The model under review builds one solid part; all positions refer to its coordinate system, in mm. A direction names the side the tool comes from. Coordinates: 2 decimals unless noted, no trailing zeros. Order: outer loops, then holes, each group sorted by start corner. A loop starts at its lowest first (then second) coordinate and runs counter-clockwise, first axis right, second up. Notation, with made-up numbers: M 23,-35.5 L 46,-35.5 A9 ccw 46,-27.5 Z; hole C 48.25,-28 d10. An arc over 180 degrees is marked long. Write each question's results on one line, items separated by ' | '.
from build123d import *

# Parameters (mm, degrees)
SKETCH1_R                 = 2.5
BOSS_EXTRUDE1_DEPTH       = 150
SKETCH3_R                 = 3
BOSS_EXTRUDE2_DEPTH       = 15
SKETCH4_R                 = 2
BOSS_EXTRUDE3_DEPTH       = 8
BOSS_EXTRUDE4_DEPTH       = 4
BOSS_EXTRUDE4_DEPTH_BACK  = 4
SKETCH5_R                 = 2.5
BOSS_EXTRUDE5_START       = 65
BOSS_EXTRUDE5_OUTLINE_R   = 4
BOSS_EXTRUDE5_OUTLINE_R_2 = 2.5
BOSS_EXTRUDE5_DEPTH       = 60


# Read off the part's stored shape, not the designer's step: Boss-Extrude5
with BuildPart() as part:
    # Sketch1 → Boss-Extrude1 (new body)
    with BuildSketch(Plane(origin=(0, 0, 0), x_dir=(0, 0, -1), z_dir=(1, 0, 0))):
        Circle(SKETCH1_R)
    extrude(amount=BOSS_EXTRUDE1_DEPTH)

    # Sketch3 → Boss-Extrude2 (add)
    with BuildSketch(Plane.ZY):
        Circle(SKETCH3_R)
    extrude(amount=BOSS_EXTRUDE2_DEPTH)

    # Sketch4 → Boss-Extrude3 (add)
    with BuildSketch(Plane(origin=(150, 0, 0), x_dir=(0, 0, -1), z_dir=(1, 0, 0))):
        Circle(SKETCH4_R)
    extrude(amount=BOSS_EXTRUDE3_DEPTH)

    # Sketch5 → Boss-Extrude4 (add, two sides: drawn at the far end of the back side and taken through both)
    with BuildSketch(Plane.XY.offset(-BOSS_EXTRUDE4_DEPTH_BACK)):
        with Locations((158, 0)):
            Circle(SKETCH5_R)
    extrude(amount=BOSS_EXTRUDE4_DEPTH + BOSS_EXTRUDE4_DEPTH_BACK)

    # Boss-Extrude5 outline → Boss-Extrude5 (add)
    with BuildSketch(Plane.YZ.offset(BOSS_EXTRUDE5_START)):
        Circle(BOSS_EXTRUDE5_OUTLINE_R)
        Circle(BOSS_EXTRUDE5_OUTLINE_R_2, mode=Mode.SUBTRACT)
    extrude(amount=BOSS_EXTRUDE5_DEPTH)


solid = part.part
1) For faces 1 (the flat face through (158, 0, -4)), 2 (the cylindrical face through (-7, 0, -3)), 3 (the flat face through (125, 2, 2)), list the 3-axis set-ups (+Z, -Z, +X, -X, +Y, -Y) from which the entire face can be reached by the end or side of a thin tool; tool diameter is ignored.
Solutions:
face 1: -Z, +X, -X, +Y, -Y | face 2: -X | face 3: none
2) Take a section at A-A on y = 0. State the section outline as (x, z) points, plus the area to 3 significant figures.
Solutions:
outline: M -15,-3 L 0,-3 L 0,-2.5 L 65,-2.5 L 65,-4 L 125,-4 L 125,-2.5 L 150,-2.5 L 150,-2 L 155.5,-2 L 155.5,-4 L 160.5,-4 L 160.5,4 L 155.5,4 L 155.5,2 L 150,2 L 150,2.5 L 125,2.5 L 125,4 L 65,4 L 65,2.5 L 0,2.5 L 0,3 L -15,3 Z | area: 1,080 mm2
3) To check wall thickness, follow line 1 along Z through (x, y) = (4, 1.5); line 2 along Y through (x, z) = (84, -0.25); line 3 along X through (y, z) = (-2, 3). State the ranges of each line that lie inside material, in increasing order.
Solutions:
line 1: -2 to 2 | line 2: -3.99 to 3.99 | line 3: 65 to 125, 156.5 to 159.5
4) The part is to be moulded in two halves that separate along X. For faces 4 (the cylindrical face through (94.58, -0.867, -3.905)), 5 (the cylindrical face through (137.32, -2.44, 0.54)), 6 (the flat face through (-15, 0, 0)), say which applies: pulls with the +X half, pulls with the -X half, needs draft (parallel to the pull), parting line crosses it, or undercut.
Solutions:
face 4: needs draft | face 5: undercut | face 6: pulls with the -X half
5) Take a section at C-C on x = 71. State the section outline as (y, z) points, plus the area to 3 significant figures.
Solutions:
outline: C 0,0 d8 | area: 50.3 mm2
6) For pin 1 (3 mm diameter, centred on y = 1, z = 1, fed in from +X); pin 2 (4 mm diameter, centred on x = 27.5, y = -2.5, fed in from +Z); pin 3 (2 mm diameter, centred on x = 137, z = -1.5, fed in from -Y); pin 4 (4 mm diameter, centred on x = 46.5, z = -2.5, fed in from +Y), all flat-tipped, find the tip position at first contact; note any pin that passes through.
Solutions:
pin 1: x = 160.5 | pin 2: z = 2.45 | pin 3: y = -2.45 | pin 4: y = 2.45
7) Take a section at B-B on x = 158. State the section outline as (y, z) points, plus the area to 3 significant figures.
Solutions:
outline: M -2.5,-4 L 2.5,-4 L 2.5,4 L -2.5,4 Z | area: 40.0 mm2
